The model under review builds one solid part; all positions refer to its coordinate system, in mm. A direction names the side the tool comes from. Coordinates: 2 decimals unless noted, no trailing zeros. Order: outer loops, then holes, each group sorted by start corner. A loop starts at its lowest first (then second) coordinate and runs counter-clockwise, first axis right, second up. Notation, with made-up numbers: (-28.5, -15.75) -> (-1.5, -15.75) arc R11 ccw to (-1.5, 2.25) -> close; hole circle Ø7 at (-10.75, 73.5). An arc over 180 degrees is marked (long way). Use one line per item in the form item = value. Start each with the question number.
(1) Take a section at D-D (z = 10). State the section outline as (x, y) points, then the cut area to 3 significant figures.
(2) Wall thickness on line 1 along X through (y, z) = (-3, 2); line 2 along X through (y, z) = (-4.5, 30.5); line 3 along Y through (x, z) = (-13, 15.5): over which ranges is each line inside the solid? List them lowest first.
(3) Insertion check: pin 1 Ø0.5 at (x, z) = (52, 5.5) entering from -Y; pin 2 Ø1.1 at (x, z) = (-51.5, 5.5) entering from +Y. Each pin has a flat end and moves straight along its axis. Give the tip position at first contact, or say it passes through.
(4) For faces 5 (the cylindrical face through (-52.4, -52.44, 17.24)), 6 (the flat face through (47.8, -31.7, 22.5)), 7 (the flat face through (-0.2, -45.5, 15)), 8 (the flat face through (52.3, 0, 7)), 9 (the flat face through (-45.3, 29, 17)), list the 3-axis set-ups (+Z, -Z, +X, -X, +Y, -Y) from which the entire face can be reached by the end or side of a thin tool; tool diameter is ignored.
(5) Take a section at C-C (z = 32.5). State the section outline as (x, y) points, then the cut area to 3 significant figures.
(6) Mouldability with a two-part tool opening along Y and no side actions: class faces 1 (the flat face through (1, 53.3, 17)), 2 (the cylindrical face through (49.888, 0.105, 9.703)), 3 (the flat face through (1, -53.3, 17)), 4 (the cylindrical face through (49.888, 0.105, 4.297)) as +Y half, -Y half, draft (parallel to the pull), parting line (faces both ways), or undercut.
```python
from build123d import *

# Parameters (mm, degrees)
SKETCH1_W            = 106.6
SKETCH1_H            = 106.6
SKETCH1_W_2          = 100.6
SKETCH1_H_2          = 100.6
BOSS_EXTRUDE1_DEPTH  = 200
SKETCH2_W            = 75
SKETCH2_H            = 10
CUT_EXTRUDE1_DEPTH   = 214.732964233
CIRPATTERN1_COUNT    = 2
CIRPATTERN1_ANGLE    = 90
FILLET1_R            = 3
BOSS_EXTRUDE2_DEPTH  = 5
SKETCH4_R            = 1.5
BOSS_EXTRUDE3_DEPTH  = 7.5
CUT_EXTRUDE3_DEPTH   = 10
FILLET2_R            = 5
FILLET2_OF_MIRROR3_R = 5
CHAMFER1_SIZE        = 5
SKETCH7_W            = 168.98996808
SKETCH7_H            = 119.087176344
TEST_PIECE_DEPTH     = 166


with BuildPart() as part:
    # Sketch1 → Boss-Extrude1 (new body)
    with BuildSketch(Plane(origin=(0, 0, 0), x_dir=(0, 1, 0), z_dir=(0, 0, 1))):
        Rectangle(SKETCH1_W, SKETCH1_H)
        Rectangle(SKETCH1_W_2, SKETCH1_H_2, mode=Mode.SUBTRACT)
    extrude(amount=BOSS_EXTRUDE1_DEPTH)

    # Sketch2 → Cut-Extrude1 (cut, symmetric)
    with BuildSketch(Plane.YZ):
        with Locations((0, 187.5)):
            Rectangle(SKETCH2_W, SKETCH2_H)
        with Locations((0, 172.5)):
            Rectangle(SKETCH2_W, SKETCH2_H)
        with Locations((0, 157.5)):
            Rectangle(SKETCH2_W, SKETCH2_H)
    cut_extrude1 = extrude(amount=CUT_EXTRUDE1_DEPTH, both=True, mode=Mode.SUBTRACT)

    # CirPattern1: Cut-Extrude1 ×2 about axis
    cirpattern1_axis = Axis((0, 0, 210), (0, 0, -1))
    for i in range(1, CIRPATTERN1_COUNT):
        add(cut_extrude1.rotate(cirpattern1_axis, i * CIRPATTERN1_ANGLE / (CIRPATTERN1_COUNT - 1)), mode=Mode.SUBTRACT)

    # Fillet1
    fillet1_edges = [part.edges().sort_by_distance(p)[0] for p in [
        (-53.3, -53.3, 100),
        (-53.3, 53.3, 100),
        (53.3, 53.3, 100),
        (53.3, -53.3, 100),
    ]]
    fillet(fillet1_edges, radius=FILLET1_R)

    # Sketch3 → Boss-Extrude2 (add)
    with BuildSketch(Plane(origin=(0, 0, 15), x_dir=(0, 1, 0), z_dir=(0, 0, 1))):
        Polygon((-50.3, -50.3), (-12.5, -50.3), (-12.5, -45.3), (-45.3, -45.3), (-45.3, 45.3), (-12.5, 45.3), (-12.5, 50.3), (-50.3, 50.3), align=None)
        Polygon((50.3, -50.3), (50.3, 50.3), (12.5, 50.3), (12.5, 45.3), (45.3, 45.3), (45.3, -45.3), (12.5, -45.3), (12.5, -50.3), align=None)
    extrude(amount=BOSS_EXTRUDE2_DEPTH)

    # Sketch4 → Boss-Extrude3 (add, symmetric)
    with BuildSketch(Plane(origin=(0, 0, 0), x_dir=(-1, 0, 0), z_dir=(0, 1, 0))):
        with Locations((49.8, 7)):
            Circle(SKETCH4_R)
    boss_extrude3 = extrude(amount=BOSS_EXTRUDE3_DEPTH, both=True)

    # Sketch6 → Cut-Extrude3 (cut, symmetric)
    with BuildSketch(Plane(origin=(0, 0, 0), x_dir=(-1, 0, 0), z_dir=(0, 1, 0))):
        Polygon((51.6, 13), (52, 13), (52.3, 12.7), (52.3, 1.3), (52, 1), (51.6, 1), (51.3, 1.3), (51.3, 12.7), align=None)
    cut_extrude3 = extrude(amount=CUT_EXTRUDE3_DEPTH, both=True, mode=Mode.SUBTRACT)

    # Fillet2
    fillet2_edges = [part.edges().sort_by_distance(p)[0] for p in [
        (-50.3, 0, 5.585786438),
        (-50.3, 0, 8.414213562),
    ]]
    fillet(fillet2_edges, radius=FILLET2_R)

    # Mirror3: Boss-Extrude3, Cut-Extrude3 across plane
    add(boss_extrude3.mirror(Plane(origin=(0, 0, 0), x_dir=(0, 0, 1), z_dir=(1, 0, 0))))
    add(cut_extrude3.mirror(Plane(origin=(0, 0, 0), x_dir=(0, 0, 1), z_dir=(1, 0, 0))), mode=Mode.SUBTRACT)

    # Fillet2 of Mirror3
    fillet2_of_mirror3_edges = [part.edges().sort_by_distance(p)[0] for p in [
        (50.3, 0, 5.585786438),
        (50.3, 0, 8.414213562),
    ]]
    fillet(fillet2_of_mirror3_edges, radius=FILLET2_OF_MIRROR3_R)

    # Chamfer1
    chamfer1_edges = [part.edges().sort_by_distance(p)[0] for p in [
        (50.3, 31.4, 20),
        (0, 50.3, 20),
        (-50.3, 31.4, 20),
        (-50.3, -31.4, 20),
        (0, -50.3, 20),
        (50.3, -31.4, 20),
    ]]
    chamfer(chamfer1_edges, length=CHAMFER1_SIZE - 0.0001)  # a hair under: the kernel refuses the full size

    # Sketch7 → test_piece (cut)
    with BuildSketch(Plane.XY.offset(200)):
        Rectangle(SKETCH7_W, SKETCH7_H)
    extrude(amount=-TEST_PIECE_DEPTH, mode=Mode.SUBTRACT)


solid = part.part
```
Findings:
q1.outline = (-53.3, -50.3) arc R3 ccw to (-50.3, -53.3) -> (50.3, -53.3) arc R3 ccw to (53.3, -50.3) -> (53.3, 50.3) arc R3 ccw to (50.3, 53.3) -> (-50.3, 53.3) arc R3 ccw to (-53.3, 50.3) -> close; hole (-52.3, -10) -> (-51.3, -10) -> (-51.3, 10) -> (-52.3, 10) -> close; hole (-50.3, -50.3) -> (50.3, -50.3) -> (50.3, -7.5) -> (50.01, -7.5) -> (50.01, 7.5) -> (50.3, 7.5) -> (50.3, 50.3) -> (-50.3, 50.3) -> (-50.3, 7.5) -> (-50.01, 7.5) -> (-50.01, -7.5) -> (-50.3, -7.5) -> close; hole (51.3, -10) -> (52.3, -10) -> (52.3, 10) -> (51.3, 10) -> close
q1.area = 1,200 mm²
q2.line_1 = -53.3 to -52.3, -51.3 to -50.3, 50.3 to 51.3, 52.3 to 53.3
q2.line_2 = -53.3 to -50.3, 50.3 to 53.3
q2.line_3 = -53.3 to -45.3, 45.3 to 53.3
q3.pin_1 = -52.93
q3.pin_2 = 53.23
q4.face_5 = +Z, -Z, -X, -Y
q4.face_6 = +Z
q4.face_7 = -Z
q4.face_8 = none
q4.face_9 = +Z, -Z
q5.outline = (-53.3, -50.3) arc R3 ccw to (-50.3, -53.3) -> (50.3, -53.3) arc R3 ccw to (53.3, -50.3) -> (53.3, 50.3) arc R3 ccw to (50.3, 53.3) -> (-50.3, 53.3) arc R3 ccw to (-53.3, 50.3) -> close; hole (-50.3, -50.3) -> (50.3, -50.3) -> (50.3, 50.3) -> (-50.3, 50.3) -> close
q5.area = 1,240 mm²
q6.face_1 = +Y half
q6.face_2 = undercut
q6.face_3 = -Y half
q6.face_4 = undercut
